The listing builds one solid part. Answer for the finished solid, in the listing's coordinates (mm). A direction names the side the tool comes from. Coordinates: 2 decimals unless noted, no trailing zeros. Loops run counter-clockwise (first coordinate to the right, second up) from the corner with the lowest first, then second, coordinate; pieces in that order, holes last. Notation, with made-up numbers: M 72,-3 L 108,-3 A17 ccw 108,10 Z; hole C 72,33.25 d5. An arc over 180 degrees is marked long. Return JSON: item names as keys, results as strings. Group by question number.
1. Section A-A (z = -7.25) is taken. Write down the section's boundary in (x, y), then the cut area to 3 significant figures.
2. Section D-D (z = 0.75) is taken. Write down the section's boundary in (x, y).
3. Which of the six approach directions +Z, -Z, +X, -X, +Y, -Y give full straight-line access (tool end or side, diameter ignored) to faces 1 (the face through (0, 33.5, -7)), 2 (the face through (-11, -26, -7)), 3 (the face through (-0.2, -31.4, -8.5))?
4. Section C-C (y = 16) is taken. Write down the section's boundary in (x, z).
5. Section B-B (z = -3.25) is taken. Write down the section's boundary in (x, y), then the cut area to 3 significant figures.
6. The mould has two halves that part along X. Classify faces 4 (the face through (-0.238, 35.598, -4.229)), 5 (the face through (0, 28, -8.989)): pulls with the +X half, pulls with the -X half, needs draft (parallel to the pull), parting line crosses it, or undercut.
7. Straight lines are drawn through the part: L1, parallel to Y at x = 8.5, z = -6; L2, parallel to Y at x = -0.5, z = 0.75; L3, parallel to Z at x = 6, y = -27.5. For each, find the intervals that lie inside material, in ascending order. Write a range as from..to.
8. Given P1, Ø12, axis at y = -27.5, z = 2.5, coming from the -X side; P2, Ø2.5, axis at x = -1, z = -8, coming from the -Y side; P3, Ø2.5, axis at x = -1, z = -6.5, coming from the +Y side; P4, Ø3, axis at x = -13.5, z = -6.5, coming from the +Y side, each flat-ended and moving along its own axis, determine where each tip first touches the part or whether it passes through.
```python
from build123d import *

# Parameters (mm, degrees)
PAD022_DEPTH    = 34
SKETCH057_W     = 3.9158892559
SKETCH057_H     = 10
POCKET030_DEPTH = 5
SKETCH058_W     = 3.9050672559
SKETCH058_H     = 9.969185
POCKET031_DEPTH = 5


with BuildPart() as part:
    # Sketch056 → Pad022 (new body)
    with BuildSketch(Plane.YZ):
        with BuildLine():
            Line((-30.5, 22.4158892559), (30.5, 22.4158892559))
            ThreePointArc((37, 15.9158892559), (35.0961940777, 20.5120833336), (30.5, 22.4158892559))
            Line((37, 15.9158892559), (37, 8.9158892559))
            ThreePointArc((33.5, 5.4158892559), (35.9748737342, 6.4410155217), (37, 8.9158892559))
            Line((33.5, 5.4158892559), (33.5, 2))
            Line((32.5, 1), (33.5, 2))
            Line((32.5, 1), (27, 1))
            Line((27, 1), (26, 2))
            Line((26, 2), (26, 5.9158892559))
            Line((26, 5.9158892559), (28.5, 5.9158892559))
            Line((28.5, 5.9158892559), (28.5, 2.5))
            Line((28.5, 2.5), (32, 2.5))
            Line((32, 2.5), (32.5, 3))
            Line((32.5, 3), (32.5, 5.9158892559))
            Line((32.5, 5.9158892559), (33.5, 5.9158892559))
            ThreePointArc((33.5, 5.9158892559), (35.6213203436, 6.7945689123), (36.5, 8.9158892559))
            Line((36.5, 15.9158892559), (36.5, 8.9158892559))
            ThreePointArc((36.5, 15.9158892559), (34.7426406871, 20.158529943), (30.5, 21.9158892559))
            Line((-30.5, 21.9158892559), (30.5, 21.9158892559))
            ThreePointArc((-30.5, 21.9158892559), (-34.7426406871, 20.158529943), (-36.5, 15.9158892559))
            Line((-36.5, 8.9158892559), (-36.5, 15.9158892559))
            ThreePointArc((-36.5, 8.9158892559), (-35.6213203436, 6.7945689123), (-33.5, 5.9158892559))
            Line((-32.5, 5.9158892559), (-33.5, 5.9158892559))
            Line((-32.5, 3), (-32.5, 5.9158892559))
            Line((-32, 2.5), (-32.5, 3))
            Line((-28.5, 2.5), (-32, 2.5))
            Line((-28.5, 5.9158892559), (-28.5, 2.5))
            Line((-26, 5.9158892559), (-28.5, 5.9158892559))
            Line((-26, 2), (-26, 5.9158892559))
            Line((-27, 1), (-26, 2))
            Line((-32.5, 1), (-27, 1))
            Line((-33.5, 2), (-32.5, 1))
            Line((-33.5, 5.4158892559), (-33.5, 2))
            ThreePointArc((-37, 8.9158892559), (-35.9748737342, 6.4410155217), (-33.5, 5.4158892559))
            Line((-37, 8.9158892559), (-37, 15.9158892559))
            ThreePointArc((-30.5, 22.4158892559), (-35.0961940777, 20.5120833336), (-37, 15.9158892559))
        make_face()
    extrude(amount=PAD022_DEPTH)

    # Sketch057 (on Face31 of Pad022) → Pocket030 (cut)
    with BuildSketch(Plane.ZX.offset(-26)):
        with Locations((3.9579446279, 17)):
            Rectangle(SKETCH057_W, SKETCH057_H)
    extrude(amount=-POCKET030_DEPTH, mode=Mode.SUBTRACT)

    # Sketch058 (on Face15 of Pocket030) → Pocket031 (cut)
    with BuildSketch(Plane(origin=(0, 26, 0), x_dir=(0, 0, -1), z_dir=(0, -1, 0))):
        with Locations((-3.9633556279, 17.0154075)):
            Rectangle(SKETCH058_W, SKETCH058_H)
    extrude(amount=-POCKET031_DEPTH, mode=Mode.SUBTRACT)


with BuildPart() as part_1:
    # Body007 placement: moved
    add(part.part.moved(Location((-17, 0, -11))))


solid = part_1.part
```
Worked out:
{
 "1": {"outline": "M -17,-33.5 L 17,-33.5 L 17,-32.5 L -17,-32.5 Z; M -17,-28.5 L -5,-28.5 L -5,-26 L -17,-26 Z; M -17,26 L -4.97,26 L -4.97,28.5 L -17,28.5 Z; M -17,32.5 L 17,32.5 L 17,33.5 L -17,33.5 Z; M 5,-28.5 L 17,-28.5 L 17,-26 L 5,-26 Z; M 5,26 L 17,26 L 17,28.5 L 5,28.5 Z", "area": "188 mm^2"},
 "2": {"outline": "M -17,-37 L 17,-37 L 17,-36.5 L -17,-36.5 Z; M -17,36.5 L 17,36.5 L 17,37 L -17,37 Z"},
 "3": {"face 1": "-Z, +X, -X, +Y", "face 2": "-Z, +X, -X", "face 3": "+X, -X"},
 "4": {"outline": "M -17,10.92 L 17,10.92 L 17,11.42 L -17,11.42 Z"},
 "5": {"outline": "M -17,-36.8 L 17,-36.8 L 17,-36.26 L -17,-36.26 Z; M -17,36.26 L 17,36.26 L 17,36.8 L -17,36.8 Z", "area": "36.4 mm^2"},
 "6": {"face 4": "needs draft", "face 5": "undercut"},
 "7": {"L1": "-33.5..-32.5, -28.5..-26, 26..28.5, 32.5..33.5", "L2": "-37..-36.5, 36.5..37", "L3": "-10..-5.08, 10.92..11.42"},
 "8": {"P1": "through", "P2": "y = -33.5", "P3": "y = 34.99", "P4": "y = 35.44"}
}
